Design review of the part built by this model. Coordinates are the model's own, in mm. Give positions to 0.01 mm unless a question says otherwise; leave off trailing zeros. Loops run counter-clockwise (first coordinate to the right, second up) from the corner with the lowest first, then second, coordinate; pieces in that order, holes last.
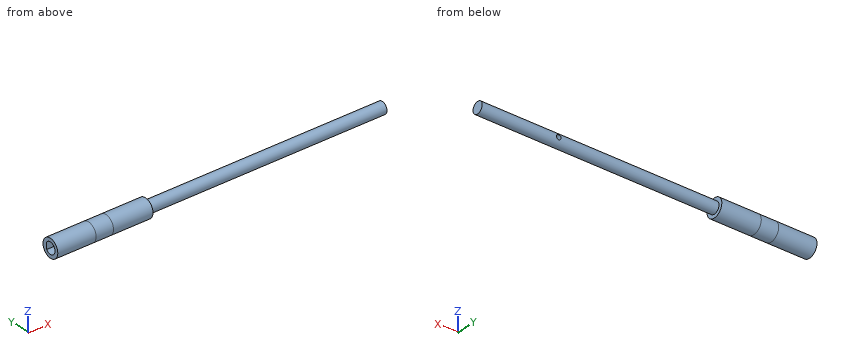
Autodesk Inventor part; units mm, degrees
ref_plane "YZ Plane" through (0, 0, 0) normal (1, 0, 0) x (0, 1, 0)
ref_plane "XZ Plane" through (0, 0, 0) normal (0, 1, 0) x (-1, 0, 0)
ref_plane "XY Plane" through (0, 0, 0) normal (0, 0, 1) x (1, 0, 0)
sketch "Sketch1" plane through (0, 0, 0) normal (1, 0, 0) x (0, 1, 0)
  circle A0 centre (0, 0) radius 4
  circle A1 centre (0, 0) radius 2.5
  line L0 (2, 0) -> (2, -1.5)
  line L1 (2, 0) -> (2, 1.5)
  dimension "d0" = 8
  dimension "d1" = 5
extrude "Extrusion1" add sketch "Sketch1" along normal blind 8 contours A0 | A1 L0 L1 picked at (2.0912, -0.8466)
sketch "Sketch2" plane through (8, 0, 0) normal (1, 0, 0) x (0, 0, -1)
  circle A0 centre (0, 0) radius 4
  circle A1 centre (0, 0) radius 2.5
extrude "Extrusion2" add sketch "Sketch2" along normal blind 2
sketch "Sketch3" plane through (8, 0, 0) normal (1, 0, 0) x (0, 0, -1)
  circle A0 centre (0, 0) radius 2.5
extrude "Extrusion3" add sketch "Sketch3" along normal blind 151
sketch "Sketch4" plane through (0, 0, 0) normal (-1, 0, 0) x (0, 0, 1)
  circle A0 centre (0, 0) radius 4
extrude "Extrusion4" cut sketch "Sketch4" against normal blind 2.5
sketch "Sketch6" plane through (0, 0, 0) normal (0, 1, 0) x (-1, 0, 0)
  line L0 (-159, 2.5) -> (-159, -2.5)
  line L1 (-159, 0) -> (-96, 0)
  circle A0 centre (-96, 0) radius 1
  point P0 (0, 0)
  dimension "d17" = 63
  dimension "d18" = 2
extrude "Extrusion6" cut sketch "Sketch6" along normal blind 10
thread "Thread2"
sketch "Sketch7" plane through (2.5, 0, 0) normal (-1, 0, 0) x (0, 0, 1)
  circle A0 centre (0, 0) radius 2.5
  circle A1 centre (0, 0) radius 4
  line L0 (1.5, 2) -> (-1.5, 2)
  line L1 (0, 2) -> (1.5, 2)
  line L2 (0, 2) -> (-1.5, 2)
extrude "Extrusion7" add sketch "Sketch7" along normal blind 16.5
sketch "Sketch8" plane through (2.5, 0, 0) normal (-1, 0, 0) x (0, 0, 1)
  circle A0 centre (0, 0) radius 2.5
  line L0 (1.5, 2) -> (-1.5, 2)
  line L1 (1.5, 2) -> (-1.5, 2)
extrude "Extrusion8" add sketch "Sketch8" along normal blind 16.5 contours L0 A0 picked at (-0.3466, 2.0912)
sketch "Sketch10" plane through (10, 0, 0) normal (1, 0, 0) x (0, 0, -1)
  circle A0 centre (0, 0) radius 2.5
  circle A1 centre (0, 0) radius 4
extrude "Extrusion9" add sketch "Sketch10" along normal blind 17
sketch "Sketch11" plane through (159, 0, 0) normal (1, 0, 0) x (0, 0, -1)
  circle A0 centre (0, 0) radius 2.5
extrude "Extrusion10" cut sketch "Sketch11" against normal blind 30
properties part number "wormgear_axis_6mm" material "Stainless Steel"
Q1. Wall thickness on line 1 (X direction, y = 0.95, z = 0); line 2 (Z direction, x = -5.5, y = 0); line 3 (Y direction, x = -3, z = 0): over which ranges is each line inside the solid? List them lowest first.
Results:
line 1: x = 8 to 95, 97 to 129
line 2: z = -4 to -2.5, 2.5 to 4
line 3: y = -4 to -2.5, 2 to 4
Q2. Take a section at A-A (x = 74). Give the boundary of the cut face in (y, z), plus the area to 3 significant figures.
Results:
outline: circle Ø5 at (0, 0)
area: 19.6 mm2
Q3. Insertion check: pin 1 (1.2 mm diameter, centred on x = 96, z = 0, fed in from -Y); pin 2 (1.6 mm diameter, centred on x = 96, z = 0, fed in from +Y); pin 3 (4 mm diameter, centred on x = 32, y = 2, fed in from +Z). Each pin has a flat end and moves straight along its axis. Give the tip position at first contact, or say it passes through.
Results:
pin 1: stops at y = -2.5
pin 2: stops at y = 0
pin 3: stops at z = 2.5
